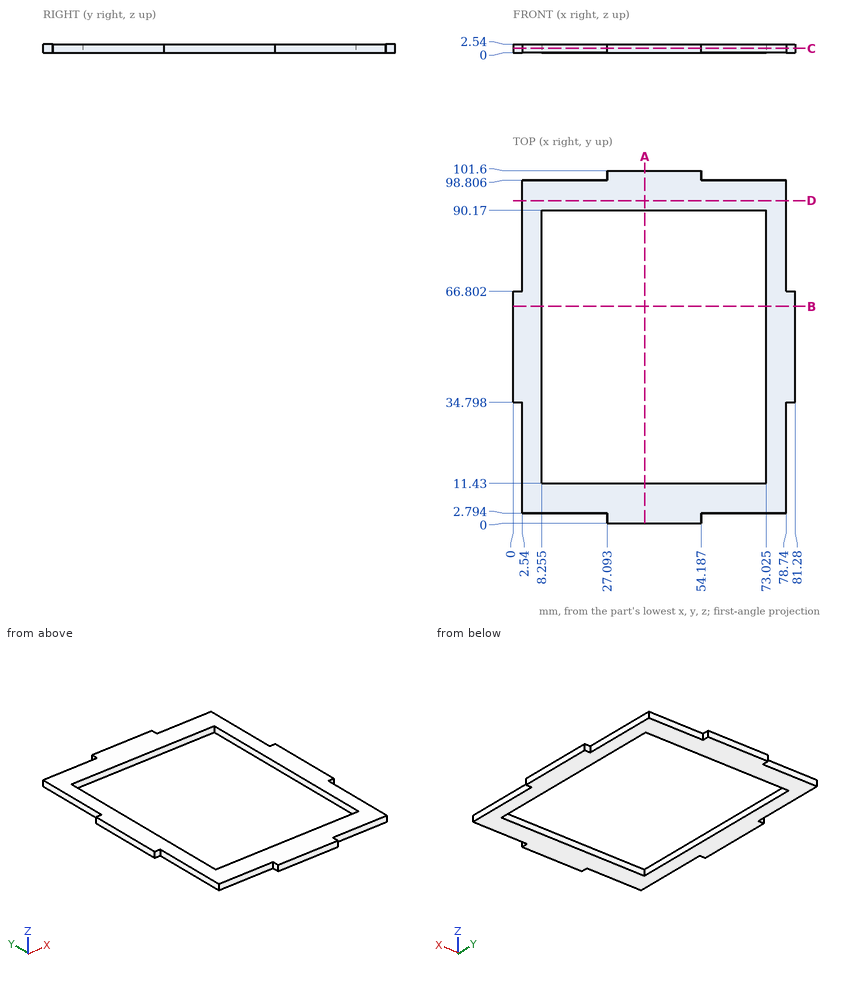
Geometry: see drawing. Coordinates: mm, zero at the bounding-box minimum. Round coordinates to 2 decimals unless told otherwise and drop trailing zeros. Write each loop counter-clockwise with the first axis right and the second up, starting at its lowest first coordinate (ties: lowest second). Pieces come first, ordered by that corner, then holes.
1) Cut plane B-B (y = 62.5). Return the cut outline in (x, z) (1 decimal).
2) Ray query, L1, parallel to Y at x = 17.5, z = 0.4; L2, parallel to X at y = 45.5, z = 0.3 (1 decimal); L3, parallel to X at y = 16, z = 2.2 (1 decimal). Return the intervals inside material, ascending.
3) Contact query for flat-ended pins moving along their axis: P1, Ø0.8, axis at y = 99.5, z = 1, coming from the +X side; P2, Ø1.3, axis at y = 100.5, z = 0.5, coming from the -X side; P3, Ø2, axis at x = 53.5, y = 14, coming from the -Z side; P4, Ø1.3, axis at y = 13, z = 1.5, coming from the -X side. Output: stop coordinate, or through.
4) Cut plane A-A (x = 38). Return the cut outline in (y, z).
5) Cut plane C-C (z = 1.25). Return the cut outline in (x, y) (1 decimal).
6) Cut plane D-D (y = 93). Return the cut outline in (x, z).
Geometry says:
1. outline: (0, 0) - (8.3, 0) - (8.3, 2.5) - (0, 2.5) - close; (73, 0) - (81.3, 0) - (81.3, 2.5) - (73, 2.5) - close
2. L1: y = 2.79 to 11.43, 90.17 to 98.81
2. L2: x = 0 to 8.3, 73 to 81.3
2. L3: x = 2.5 to 8.3, 73 to 78.7
3. P1: stops at x = 54.19
3. P2: stops at x = 27.09
3. P3: passes through
3. P4: stops at x = 2.54
4. outline: (0, 0) - (11.43, 0) - (11.43, 2.54) - (0, 2.54) - close; (90.17, 0) - (101.6, 0) - (101.6, 2.54) - (90.17, 2.54) - close
5. outline: (0, 34.8) - (2.5, 34.8) - (2.5, 2.8) - (27.1, 2.8) - (27.1, 0) - (54.2, 0) - (54.2, 2.8) - (78.7, 2.8) - (78.7, 34.8) - (81.3, 34.8) - (81.3, 66.8) - (78.7, 66.8) - (78.7, 98.8) - (54.2, 98.8) - (54.2, 101.6) - (27.1, 101.6) - (27.1, 98.8) - (2.5, 98.8) - (2.5, 66.8) - (0, 66.8) - close; hole (8.3, 11.4) - (73, 11.4) - (73, 90.2) - (8.3, 90.2) - close
6. outline: (2.54, 0) - (78.74, 0) - (78.74, 2.54) - (2.54, 2.54) - close
